Autodesk Inventor part; units mm, degrees
ref_plane "YZ Plane" through (0, 0, 0) normal (1, 0, 0) x (0, 1, 0)
ref_plane "XZ Plane" through (0, 0, 0) normal (0, 1, 0) x (-1, 0, 0)
ref_plane "XY Plane" through (0, 0, 0) normal (0, 0, 1) x (1, 0, 0)
sketch "Sketch1" plane through (0, 0, 0) normal (1, 0, 0) x (0, 1, 0)
  circle A0 centre (0, 0) radius 6
  line L0 (-30, -40) -> (9.8205, -22.9904)
  line L1 (-30, 40) -> (9.8205, 22.9904)
  line L2 (-33, -35) -> (-30, -35)
  line L3 (-33, 35) -> (-30, 35)
  line L4 (-46, 35) -> (-46, -35) construction
  line L5 (-30, 35) -> (-30, 40)
  line L6 (-30, -35) -> (-30, -40)
  line L7 (-43, 35) -> (-46, 35)
  arc A1 (9.8205, -22.9904) -> (9.8205, 22.9904) centre (0, 0) ccw
  circle A2 centre (6.4234, 7.75) radius 1.5
  circle A3 centre (6.4234, -7.75) radius 1.5
  circle A4 centre (-7, -15.5) radius 1.5
  circle A5 centre (-20.4234, -7.75) radius 1.5
  circle A6 centre (-20.4234, 7.75) radius 1.5
  circle A7 centre (-7, 15.5) radius 1.5
  line L8 (-46, -35) -> (-43, -35)
  line L9 (-43, -35) -> (-43, -32)
  line L10 (-43, -32) -> (-33, -32)
  line L11 (-33, -32) -> (-33, -35)
  line L12 (-43, 35) -> (-43, 32)
  line L13 (-43, 32) -> (-33, 32)
  line L14 (-33, 32) -> (-33, 35)
  line L15 (-46, 35) -> (-53, 35)
  line L16 (-53, 35) -> (-53, -35)
  line L17 (-53, -35) -> (-46, -35)
  point P0 (-46, 0)
  dimension "d0" = 12
  dimension "d40" = 70
  dimension "d58" = 25
  dimension "d59" = 5
  dimension "d61" = 39.8205
  dimension "d62" = 17.0096
  dimension "d63" = 39.8205
  dimension "d68" = 80
  dimension "d70" = 46
  dimension "d76" = 9.8205
  dimension "d79" = 3
  dimension "d80" = 3
  dimension "d81" = 3
  dimension "d82" = 3
  dimension "d83" = 3
  dimension "d84" = 3
  dimension "d89" = 7
  dimension "d90" = 7
  dimension "d91" = 15.5
  dimension "d92" = 15.5
  dimension "d93" = 7.75
  dimension "d94" = 7.75
  dimension "d95" = 20.4234
  dimension "d96" = 20.4234
  dimension "d97" = 7.75
  dimension "d98" = 7.75
  dimension "d99" = 6.4234
  dimension "d100" = 6.4234
  dimension "d105" = 3
  dimension "d108" = 3
  dimension "d112" = 3
  dimension "d113" = 5
  dimension "d116" = 3
  dimension "d117" = 3
  dimension "d118" = 10
  dimension "d119" = 3
  dimension "d120" = 3
  dimension "d121" = 10
  dimension "d122" = 3
  dimension "d123" = 7
  dimension "d124" = 70
  dimension "d125" = 7
extrude "Extrusion1" add sketch "Sketch1" along normal blind 3
properties part number "baseSoporte3" material "PMMA Plastic"
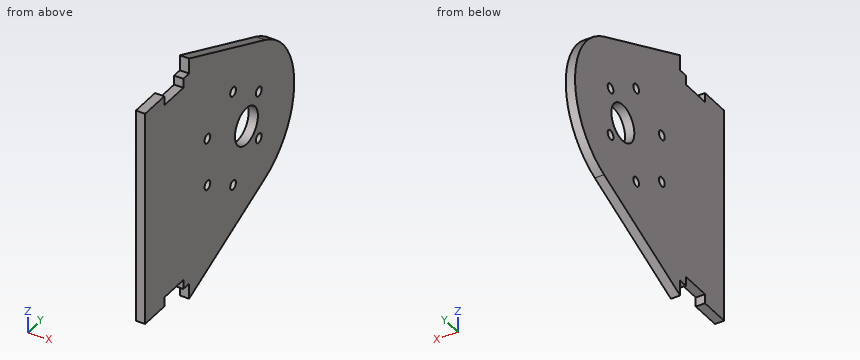
Geometry check sheet. Reference: the model listing, model coordinates, mm. Give positions to 0.01 mm unless a question says otherwise; leave off trailing zeros. Write each loop counter-clockwise with the first axis right and the second up, starting at its lowest first coordinate (ties: lowest second). Pieces come first, ordered by that corner, then holes. Notation, with made-up numbers: M 73,85 L 79,85 A13 cw 79,90 Z; hole C -39,86.5 d7. An arc over 180 degrees is marked long. Answer as CSV lines item,"result". Start each with the question number.
Q1. Section check C-C, the plane x = 1. Record the cut outline in (y, z).
Q2. Go/stop test with flat-tipped pins: pin 1 (1 mm diameter, centred on x = 2, y = -34.5, fed in from -Z); pin 2 (1.5 mm diameter, centred on x = 2, y = -32, fed in from +Z); pin 3 (0.9 mm diameter, centred on x = 1, z = -33.5, fed in from +Y). Record where each tip stops, or that it passes through.
Q3. Material ranges on L1, parallel to Y at x = 1.65, z = -6.5; L2, parallel to Z at x = 0.8, y = -20; L3, parallel to Z at x = 0.25, y = 2, recorded low to high.
Q4. Section check D-D, the plane z = -22. Record the cut outline in (x, y).
Q5. Section check B-B, the plane y = 0.5. Record the cut outline in (x, z).
Q6. Section check A-A, the plane z = 0. Record the cut outline in (x, y).
Geometry says:
1,outline,"M -53,-35 L -43,-35 L -43,-32 L -33,-32 L -33,-35 L -30,-35 L -30,-40 L 9.82,-22.99 A25 ccw 9.82,22.99 L -30,40 L -30,35 L -33,35 L -33,32 L -43,32 L -43,35 L -53,35 Z; hole C -20.42,-7.75 d3; hole C -20.42,7.75 d3; hole C -7,-15.5 d3; hole C -7,15.5 d3; hole C 0,0 d12; hole C 6.42,-7.75 d3; hole C 6.42,7.75 d3"
2,pin 1,"z = -32"
2,pin 2,"z = 35"
2,pin 3,"y = -13.73"
3,L1,"-53 to -21.25, -19.59 to 5.59, 7.25 to 24.14"
3,L2,"-35.73 to -9.19, -6.31 to 6.31, 9.19 to 35.73"
3,L3,"-26.33 to -5.66, 5.66 to 26.33"
4,outline,"M 0,-53 L 3,-53 L 3,11.87 L 0,11.87 Z"
5,outline,"M 0,-26.97 L 3,-26.97 L 3,-5.98 L 0,-5.98 Z; M 0,5.98 L 3,5.98 L 3,26.97 L 0,26.97 Z"
6,outline,"M 0,-53 L 3,-53 L 3,-6 L 0,-6 Z; M 0,6 L 3,6 L 3,25 L 0,25 Z"
